Verification items for the finished model (mm, model axes). A direction names the side the tool comes from. Give positions to 0.01 mm unless a question says otherwise; leave off trailing zeros. Loops run counter-clockwise (first coordinate to the right, second up) from the corner with the lowest first, then second, coordinate; pieces in that order, holes last. Notation, with made-up numbers: (29.25, -33) -> (80.25, -33) arc R25 cw to (80.25, -17) -> close; hole circle Ø7 at (54, -1). An arc over 180 degrees is marked (long way). Answer in a Markdown table with one row per item. Add a question column.
Q1. Material ranges on probe 1 along Y at (x, z) = (20, 3); probe 2 along Z at (x, y) = (17, -12); probe 3 along Y at (x, z) = (20, 5.5), recorded low to high.
Q2. Section check B-B on y = -12. Enter the section's corners in (x, z).
Q3. Section check A-A on z = 1.5. Enter the section's corners in (x, y).
Q4. Release check for a two-part mould opening along Y. For faces 1 (the face through (49.37, 5.41, 3.82)), 2 (the face through (39.235, 22.329, 5.066)), 3 (the face through (20, 38.141, 5)) record: pulls with the +Y half, pulls with the -Y half, needs draft (parallel to the pull), parting line crosses it, or undercut.
Q5. Section check D-D on y = 13.5. Give the number of separate pieces and of enclosed holes in the cut face, and give its area (3 significant figures).
Q6. Set-up check for faces 4 (the face through (24, 8, 7)), 5 (the face through (44.86, 25.58, 4.93)), 6 (the face through (0, -10.8, 3.8)), 7 (the face through (40, -10.8, 3.8)), 8 (the face through (29.37, 40.05, 3.82)): record each of +Z, -Z, +X, -X, +Y, -Y from which the full face is reachable in a straight line by a thin tool's end or side.
Q7. Section check C-C on x = 17. Enter the section's corners in (y, z).
Q8. Gauge pin test, flat ends, axial feed: P1, Ø3, axis at y = -9.5, z = 6.5, coming from the +X side; P2, Ø2, axis at x = 30, z = 8.5, coming from the +Y side; P3, Ø5, axis at y = -11, z = 6, coming from the -X side. Record the tip position at first contact, or that the pin passes through.
```python
from build123d import *

# Parameters (mm, degrees)
F1_DEPTH  = 10
F2_DEPTH  = 17
F3_DEPTH  = 17
F4_DEPTH  = 17
F5_R      = 4.5
F6_DEPTH  = 25
F7_DEPTH  = 3
F8_SIZE   = 7
F9_R      = 1.5
F10_DEPTH = 45.3
F11_R     = 1.5
F12_DEPTH = 40
F13_R     = 1.5
F14_DEPTH = 40


with BuildPart() as f1:
    # F0 (on Top) → F1 (new body)
    with BuildSketch(Plane.XY):
        Polygon((20, 34.6410161514), (0, 0), (40, 0), align=None)
    extrude(amount=F1_DEPTH)

    # F2 (add): a face of the model
    f2_faces = [f1.faces().sort_by_distance(p)[0] for p in [
        (10, 17.3205080757, 5),
    ]]
    extrude(f2_faces, amount=F2_DEPTH)

    # F3 (add): a face of the model
    f3_faces = [f1.faces().sort_by_distance(p)[0] for p in [
        (30, 17.3205080757, 5),
    ]]
    extrude(f3_faces, amount=F3_DEPTH)

    # F4 (add): a face of the model
    f4_faces = [f1.faces().sort_by_distance(p)[0] for p in [
        (20, 0, 5),
    ]]
    extrude(f4_faces, amount=F4_DEPTH)

    # F5 (on face) → F6 (cut)
    with BuildSketch(Plane.XY.offset(10)):
        with BuildLine():
            ThreePointArc((9.525644347, 18.5470053838), (8.3026957714, 20.1407829972), (6.4467024308, 19.3720053838))
            ThreePointArc((6.4467024308, 19.3720053838), (7.050644347, 17.1180634675), (9.3045862633, 17.7220053838))
            ThreePointArc((9.3045862633, 17.7220053838), (9.4694219604, 18.1199539594), (9.525644347, 18.5470053838))
        make_face()
        with BuildLine():
            ThreePointArc((21.65, 25.5470053838), (21.166726189, 26.7137315728), (20, 27.1970053838))
            ThreePointArc((20, 27.1970053838), (18.833273811, 24.3802791948), (21.65, 25.5470053838))
        make_face()
        with BuildLine():
            ThreePointArc((33.774355653, 18.5470053838), (33.7181332664, 18.9740568082), (33.5532975692, 19.3720053838))
            ThreePointArc((33.5532975692, 19.3720053838), (31.299355653, 19.9759473), (30.6954137367, 17.7220053838))
            ThreePointArc((30.6954137367, 17.7220053838), (32.5514070774, 16.9532277704), (33.774355653, 18.5470053838))
        make_face()
        with BuildLine():
            ThreePointArc((30.6954137367, 5.3720053838), (31.299355653, 3.1180634675), (33.5532975692, 3.7220053838))
            ThreePointArc((33.5532975692, 3.7220053838), (33.7181332664, 4.1199539594), (33.774355653, 4.5470053838))
            ThreePointArc((33.774355653, 4.5470053838), (32.5514070774, 6.1407829972), (30.6954137367, 5.3720053838))
        make_face()
        with BuildLine():
            ThreePointArc((20, -0.8029946162), (18.35, -2.4529946162), (20, -4.1029946162))
            ThreePointArc((20, -4.1029946162), (21.166726189, -3.6197208052), (21.65, -2.4529946162))
            ThreePointArc((21.65, -2.4529946162), (21.166726189, -1.2862684272), (20, -0.8029946162))
        make_face()
        with BuildLine():
            ThreePointArc((9.3045862633, 5.3720053838), (7.050644347, 5.9759473), (6.4467024308, 3.7220053838))
            ThreePointArc((6.4467024308, 3.7220053838), (8.3026957714, 2.9532277704), (9.525644347, 4.5470053838))
            ThreePointArc((9.525644347, 4.5470053838), (9.4694219604, 4.9740568082), (9.3045862633, 5.3720053838))
        make_face()
        with Locations((20, 11.5470053838)):
            Circle(F5_R)
    extrude(amount=-F6_DEPTH, mode=Mode.SUBTRACT)

    # F5 (on face) → F7 (cut)
    with BuildSketch(Plane.XY.offset(10)):
        with BuildLine():
            ThreePointArc((28.5, 11.5470053838), (28.2103695235, 13.7469672672), (27.3612159322, 15.7970053838))
            ThreePointArc((27.3612159322, 15.7970053838), (20, 20.0470053838), (12.6387840678, 15.7970053838))
            ThreePointArc((12.6387840678, 15.7970053838), (11.5, 11.5470053838), (12.6387840678, 7.2970053838))
            ThreePointArc((12.6387840678, 7.2970053838), (15.75, 4.1857894516), (20, 3.0470053838))
            ThreePointArc((20, 3.0470053838), (24.25, 4.1857894516), (27.3612159322, 7.2970053838))
            ThreePointArc((27.3612159322, 7.2970053838), (28.2103695235, 9.3470435004), (28.5, 11.5470053838))
        make_face()
        with Locations((20, 11.5470053838)):
            Circle(F5_R, mode=Mode.SUBTRACT)
    extrude(amount=-F7_DEPTH, mode=Mode.SUBTRACT)

    # F8
    f8_edges = [f1.edges().sort_by_distance(p)[0] for p in [
        (0, 0, 5),
        (40, 0, 5),
        (20, 34.641016, 5),
    ]]
    chamfer(f8_edges, length=F8_SIZE)

    # F9 (on face) → F10 (cut)
    with BuildSketch(Plane(origin=(0, 0, 0), x_dir=(0.8660254038, -0.5, 0), z_dir=(-0.5, -0.8660254038, 0))):
        with Locations((-12, 5)):
            Circle(F9_R)
    extrude(amount=-F10_DEPTH, mode=Mode.SUBTRACT)

    # F11 (on face) → F12 (cut)
    with BuildSketch(Plane(origin=(0, 0, 0), x_dir=(0, -1, 0), z_dir=(-1, 0, 0))):
        with Locations((12, 5)):
            Circle(F11_R)
    extrude(amount=-F12_DEPTH, mode=Mode.SUBTRACT)

    # F13 (on face) → F14 (cut)
    with BuildSketch(Plane(origin=(10, -17.3205080757, 0), x_dir=(0.8660254038, 0.5, 0), z_dir=(0.5, -0.8660254038, 0))):
        with Locations((46.6410161514, 5)):
            Circle(F13_R)
    extrude(amount=-F14_DEPTH, mode=Mode.SUBTRACT)


solid = f1.part
```
Taken from the geometry:
| question | item | result |
|---|---|---|
| 1 | probe 1 | y = -17 to -4.1, -0.8 to 7.05, 16.05 to 23.9, 27.2 to 38.14 |
| 1 | probe 2 | z = 0 to 3.5, 6.5 to 10 |
| 1 | probe 3 | y = -17 to -13.41, -10.59 to -4.1, -0.8 to 7.05, 16.05 to 23.9, 27.2 to 38.14 |
| 2 | outline | (0, 0) -> (40, 0) -> (40, 3.5) -> (0, 3.5) -> close; (0, 6.5) -> (40, 6.5) -> (40, 10) -> (0, 10) -> close |
| 3 | outline | (-14.72, 8.5) -> (-6.06, 3.5) -> (0, -7) -> (0, -17) -> (40, -17) -> (40, -7) -> (46.06, 3.5) -> (54.72, 8.5) -> (34.72, 43.14) -> (26.06, 38.14) -> (13.94, 38.14) -> (5.28, 43.14) -> close; hole circle Ø3.3 at (7.88, 4.55); hole circle Ø3.3 at (7.88, 18.55); hole circle Ø9 at (20, 11.55); hole circle Ø3.3 at (20, -2.45); hole circle Ø3.3 at (20, 25.55); hole circle Ø3.3 at (32.12, 4.55); hole circle Ø3.3 at (32.12, 18.55) |
| 4 | face 1 | pulls with the -Y half |
| 4 | face 2 | undercut |
| 4 | face 3 | pulls with the +Y half |
| 5 | separate pieces | 2 |
| 5 | enclosed holes | 2 |
| 5 | area | 514 mm² |
| 6 | face 4 | +Z |
| 6 | face 5 | +Z, -Z, +X, +Y |
| 6 | face 6 | +Z, -Z, -X, -Y |
| 6 | face 7 | +Z, -Z, +X, -Y |
| 6 | face 8 | +Z, -Z, +Y |
| 7 | outline | (-17, 0) -> (8.19, 0) -> (8.19, 7) -> (3.59, 7) -> (3.59, 10) -> (-17, 10) -> close; (14.9, 0) -> (38.14, 0) -> (38.14, 10) -> (19.5, 10) -> (19.5, 7) -> (14.9, 7) -> close; hole circle Ø3 at (-12, 5) |
| 8 | P1 | stops at x = 40 |
| 8 | P2 | stops at y = 40.99 |
| 8 | P3 | stops at x = 0 |
